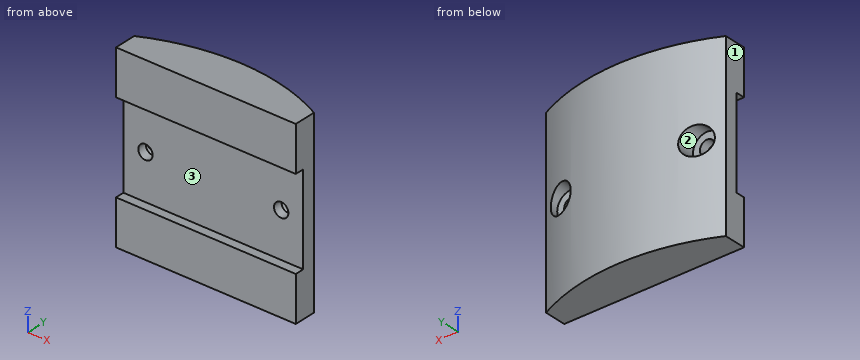
```python
from build123d import *

# Parameters (mm, degrees)
RESSALTO_EXTRUS_O1_DEPTH   = 40
ESBO_O2_R                  = 1.6
CORTE_EXTRUS_O1_DEPTH      = 2
CORTE_EXTRUS_O2_REACH      = 47.069
CORTE_EXTRUS_O2_END_RADIUS = 45
ESBO_O3_R                  = 3.15
ESBO_O4_W                  = 40
ESBO_O4_H                  = 10
RESSALTO_EXTRUS_O2_DEPTH   = 2


with BuildPart() as part:
    # Esboço1 → Ressalto-extrusão1 (new body)
    with BuildSketch(Plane.XY):
        with BuildLine():
            Line((-20, 40.311288741), (-20, 37.411288741))
            Line((-20, 37.411288741), (20, 37.411288741))
            Line((20, 37.411288741), (20, 40.311288741))
            ThreePointArc((20, 40.311288741), (0, 45), (-20, 40.311288741))
        make_face()
    extrude(amount=RESSALTO_EXTRUS_O1_DEPTH)

    # Esboço2 → Corte-extrusão1 (cut)
    with BuildSketch(Plane.XZ.offset(-37.411288741)):
        with Locations(Location((15.1, 20, 0), (0, 0, 270))):
            Circle(ESBO_O2_R)
        with Locations(Location((-15.1, 20, 0), (0, 0, 270))):
            Circle(ESBO_O2_R)
    extrude(amount=-CORTE_EXTRUS_O1_DEPTH, mode=Mode.SUBTRACT)

    # Corte-extrusão2: up to this cylinder (the profile starts inside it)
    corte_extrus_o2_end = Plane(origin=(0, 0, 20), z_dir=(0, 0, -1)) * Cylinder(CORTE_EXTRUS_O2_END_RADIUS, 185.138, mode=Mode.PRIVATE)
    # Esboço3 → Corte-extrusão2 (cut, up to the surface)
    with BuildSketch(Plane.XZ.offset(-39.411288741), mode=Mode.PRIVATE) as corte_extrus_o2_sk1:
        with Locations(Location((15.1, 20, 0), (0, 0, 270))):
            Circle(ESBO_O3_R)
    corte_extrus_o2_tool1 = extrude(corte_extrus_o2_sk1.sketch, amount=-CORTE_EXTRUS_O2_REACH, mode=Mode.PRIVATE) & corte_extrus_o2_end
    add(corte_extrus_o2_tool1.solids().sort_by_distance((15.1, 39.411289, 20))[0], mode=Mode.SUBTRACT)
    # Esboço3 → Corte-extrusão2 (cut, up to the surface)
    with BuildSketch(Plane.XZ.offset(-39.411288741), mode=Mode.PRIVATE) as corte_extrus_o2_sk2:
        with Locations(Location((-15.1, 20, 0), (0, 0, 270))):
            Circle(ESBO_O3_R)
    corte_extrus_o2_tool2 = extrude(corte_extrus_o2_sk2.sketch, amount=-CORTE_EXTRUS_O2_REACH, mode=Mode.PRIVATE) & corte_extrus_o2_end
    add(corte_extrus_o2_tool2.solids().sort_by_distance((-15.1, 39.411289, 20))[0], mode=Mode.SUBTRACT)

    # Esboço4 → Ressalto-extrusão2 (add)
    with BuildSketch(Plane.XZ.offset(-37.411288741)):
        with Locations((0, 35)):
            Rectangle(ESBO_O4_W, ESBO_O4_H)
        with Locations((0, 5)):
            Rectangle(ESBO_O4_W, ESBO_O4_H)
    extrude(amount=RESSALTO_EXTRUS_O2_DEPTH)


solid = part.part
```
Verification items for the finished model (mm, model axes). Face numbers are marked on the shaded views. A direction names the side the tool comes from. Coordinates: 2 decimals unless noted, no trailing zeros. Loops run counter-clockwise (first coordinate to the right, second up) from the corner with the lowest first, then second, coordinate; pieces in that order, holes last. Notation, with made-up numbers: (50.25, 14) -> (71.25, 14) arc R19 cw to (71.25, 32) -> close; hole circle Ø4 at (34, 73.25). An arc over 180 degrees is marked (long way). Answer in a Markdown table with one row per item. Add a question column.
1. Section check C-C, the plane x = 9. Enter the section's corners in (y, z), then the cut area to 3 significant figures.
2. Depth check by flat-ended pin: P1, Ø7, axis at x = -14.5, z = 18.5, coming from the +Y side; P2, Ø5, axis at x = 15.1, z = 20, coming from the +Y side; P3, Ø2, axis at y = 42, z = 9, coming from the -X side. Enter the tip coordinate at first touch or a pass-through.
3. Section check B-B, the plane z = 15. Enter the section's corners in (x, y).
4. Access from +Z, -Z, +X, -X, +Y, -Y to the whole of each face (thin tool, end or side, straight path). Record for the marked faces 1, 2 and 3.
5. Material ranges on probe 1 along X at (y, z) = (38.15, 20); probe 2 along X at (y, z) = (40.85, 20); probe 3 along Z at (x, y) = (15.1, 42.05), recorded low to high. Write a range as [from, to].
6. Section check A-A, the plane x = 15.1. Enter the section's corners in (y, z), then the cut area to 3 significant figures.
7. Section check D-D, the plane y = 44. Enter the section's corners in (x, z).
Derived:
| question | item | result |
|---|---|---|
| 1 | outline | (35.41, 0) -> (44.09, 0) -> (44.09, 40) -> (35.41, 40) -> (35.41, 30) -> (37.41, 30) -> (37.41, 10) -> (35.41, 10) -> close |
| 1 | area | 307 mm² |
| 2 | P1 | stops at y = 43.63 |
| 2 | P2 | stops at y = 39.41 |
| 2 | P3 | stops at x = -18.55 |
| 3 | outline | (-20, 37.41) -> (20, 37.41) -> (20, 40.31) arc R45 ccw to (-20, 40.31) -> close |
| 4 | face 1 | +Z, -Z, -X, +Y, -Y |
| 4 | face 2 | +Y |
| 4 | face 3 | +X, -X, -Y |
| 5 | probe 1 | x = [-20, -16.7], [-13.5, 13.5], [16.7, 20] |
| 5 | probe 2 | x = [-18.88, -18.25], [-11.95, 11.95], [18.25, 18.88] |
| 5 | probe 3 | z = [0, 16.85], [23.15, 40] |
| 6 | outline | (35.41, 0) -> (42.39, 0) -> (42.39, 16.85) -> (39.41, 16.85) -> (39.41, 18.4) -> (37.41, 18.4) -> (37.41, 10) -> (35.41, 10) -> close; (35.41, 30) -> (37.41, 30) -> (37.41, 21.6) -> (39.41, 21.6) -> (39.41, 23.15) -> (42.39, 23.15) -> (42.39, 40) -> (35.41, 40) -> close |
| 6 | area | 214 mm² |
| 7 | outline | (-9.43, 0) -> (9.43, 0) -> (9.43, 40) -> (-9.43, 40) -> close |
